Geometry check sheet. Reference: the model listing, model coordinates, mm. A direction names the side the tool comes from. Round coordinates to 2 decimals unless told otherwise and drop trailing zeros. Order: outer loops, then holes, each group sorted by start corner. A loop starts at its lowest first (then second) coordinate and runs counter-clockwise, first axis right, second up. Notation, with made-up numbers: (16, -19.75) -> (66, -19.75) arc R21 cw to (66, 5.25) -> close; hole circle Ø4 at (41, 24). An arc over 180 degrees is marked (long way). Use a Markdown table: item, result. Add a question column.
Item 1: Gauge pin test, flat ends, axial feed: pin 1 Ø3 at (x, z) = (12.5, -0.5) entering from -Y; pin 2 Ø4 at (y, z) = (12, -1) entering from -X; pin 3 Ø2 at (x, y) = (-5, 10.5) entering from +Z. Record the tip position at first contact, or that the pin passes through.
Item 2: Sectioned sample at C-C, the plane z = 1. Record the cut outline in (x, y), and give its area (3 significant figures).
Item 3: Material ranges on probe 1 along Y at (x, z) = (0, 2.95); probe 2 along X at (y, z) = (-7.5, 2.75); probe 3 along Y at (x, z) = (0, -3.05), recorded low to high. Write a range as [from, to].
Item 4: Mould release check, pull along X, two halves, no side actions. Record for faces 1 (the flat face through (9.3, -9.3, -3.5)), 2 (the cylindrical face through (9.139, 14.334, -3.007)), 3 (the cylindrical face through (-4.01, -18.06, -0.04)): pulls with the +X half, pulls with the -X half, needs draft (parallel to the pull), parting line crosses it, or undercut.
Item 5: Set-up check for faces 4 (the flat face through (16, -7, 3.5)), 5 (the cylindrical face through (12.932, -5.362, 3.007)), 6 (the flat face through (-6, 13, -2.5)): record each of +Z, -Z, +X, -X, +Y, -Y from which the full face is reachable in a straight line by a thin tool's end or side.
from build123d import *

# Parameters (mm, degrees)
AUFSATZ_LINEAR_AUSTRAGEN1_DEPTH      = 3.5
AUFSATZ_LINEAR_AUSTRAGEN1_DEPTH_BACK = 3.5
SKIZZE1_R                            = 18.5
SKIZZE1_R_2                          = 12.5
SKIZZE2_R                            = 17
SKIZZE2_R_2                          = 14
SCHNITT_LINEAR_AUSTRAGEN1_DEPTH      = 1
FASE1_SIZE                           = 0.5


with BuildPart() as part:
    # Skizze1 → Aufsatz-Linear austragen1 (new, two sides: drawn at the far end of the back side and taken through both)
    with BuildSketch(Plane.XY.offset(-AUFSATZ_LINEAR_AUSTRAGEN1_DEPTH_BACK)):
        Circle(SKIZZE1_R)
        Circle(SKIZZE1_R_2, mode=Mode.SUBTRACT)
    extrude(amount=AUFSATZ_LINEAR_AUSTRAGEN1_DEPTH + AUFSATZ_LINEAR_AUSTRAGEN1_DEPTH_BACK)

    # Skizze2 → Schnitt-Linear austragen1 (cut)
    with BuildSketch(Plane.XY.offset(3.5)):
        Circle(SKIZZE2_R)
        Circle(SKIZZE2_R_2, mode=Mode.SUBTRACT)
    schnitt_linear_austragen1 = extrude(amount=-SCHNITT_LINEAR_AUSTRAGEN1_DEPTH, mode=Mode.SUBTRACT)

    # Spiegeln1: Schnitt-Linear austragen1 across plane
    add(schnitt_linear_austragen1.mirror(Plane.XY), mode=Mode.SUBTRACT)

    # Fase1
    fase1_edges = [part.edges().sort_by_distance(p)[0] for p in [
        (-18.5, 0, -3.5),
        (-12.5, 0, -3.5),
        (-18.5, 0, 3.5),
        (-12.5, 0, 3.5),
    ]]
    chamfer(fase1_edges, length=FASE1_SIZE)


solid = part.part
Found:
| question | item | result |
|---|---|---|
| 1 | pin 1 | stops at y = -14.87 |
| 1 | pin 2 | stops at x = -15.56 |
| 1 | pin 3 | stops at z = 3.13 |
| 2 | outline | circle Ø37 at (0, 0); hole circle Ø25 at (0, 0) |
| 2 | area | 584 mm2 |
| 3 | probe 1 | y = [-18.5, -17], [-14, -12.5], [12.5, 14], [17, 18.5] |
| 3 | probe 2 | x = [-16.91, -15.26], [-11.82, -10], [10, 11.82], [15.26, 16.91] |
| 3 | probe 3 | y = [-18.45, -17], [-14, -12.55], [12.55, 14], [17, 18.45] |
| 4 | face 1 | needs draft |
| 4 | face 2 | undercut |
| 4 | face 3 | parting line crosses it |
| 5 | face 4 | +Z, +X, -X, +Y, -Y |
| 5 | face 5 | +Z |
| 5 | face 6 | -Z |
